Job drawing, mm, ordinate dimensions from the low corner. One solid piece. Give positions to 0.01 mm unless a question says otherwise; leave off trailing zeros. Order: outer loops, then holes, each group sorted by start corner. A loop starts at its lowest first (then second) coordinate and runs counter-clockwise, first axis right, second up. Notation, with made-up numbers: (35.25, 13.25) -> (85.25, 13.25) arc R6 cw to (85.25, 17.25) -> close; hole circle Ø11 at (75, 60.5). An arc over 180 degrees is marked (long way). Write item = value, one per line. Start each with the question number.
(1) Saw through at B-B, the plane x = 110.5. List the corners of the cut face in (y, z), then the cut area to 3 significant figures.
(2) Two-plate mould, pull along Y, no slides. Class the marked faces 1 and 2: pulls with the +Y half, pulls with the -Y half, needs draft (parallel to the pull), parting line crosses it, or undercut.
(3) Saw through at A-A, the plane y = 20.5. List the corners of the cut face in (x, z).
(4) Probe line 1 along Y through (x, z) = (131.5, 63.5); line 2 along Z through (x, y) = (230, 13.5). List the from-to ranges inside material, lowest first. Write a range as from..to.
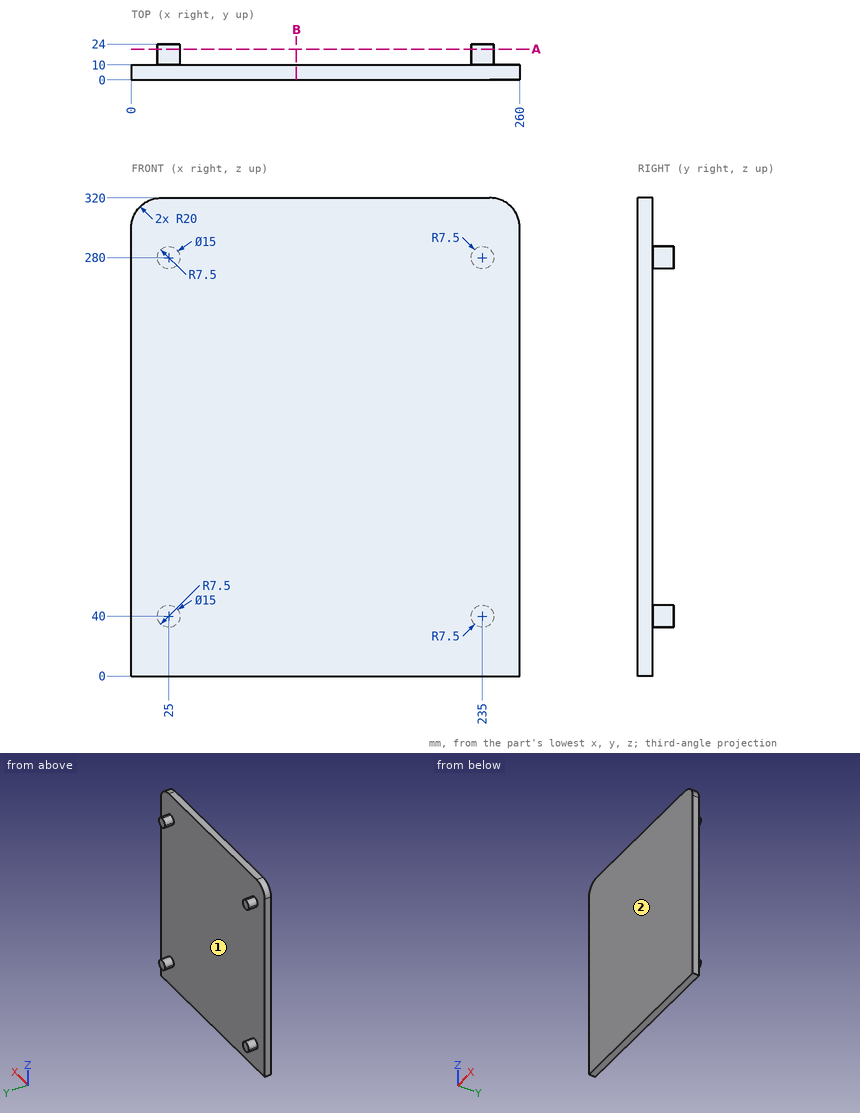
Results list:
q1.outline = (0, 0) -> (10, 0) -> (10, 320) -> (0, 320) -> close
q1.area = 3,200 mm^2
q2.face_1 = pulls with the +Y half
q2.face_2 = pulls with the -Y half
q3.outline = circle Ø15 at (25, 40); circle Ø15 at (25, 280); circle Ø15 at (235, 40); circle Ø15 at (235, 280)
q4.line_1 = 0..10
q4.line_2 = 34.41..45.59, 274.41..285.59
